```python
from build123d import *

# Parameters (mm, degrees)
ESQUISSE1_W                     = 250
ESQUISSE1_H                     = 400
BOSS_EXTRU_1_DEPTH              = 10
ESQUISSE2_R                     = 13.5
ENL_V_MAT_EXTRU_1_DEPTH         = 237.061432682
CHANFREIN1_SIZE                 = 3
TROU_TARAUD_M51_D               = 4.2
TROUS_DE_CENTRAGE_4_0MM2_D      = 4
TROUS_DE_CENTRAGE_6_0MM2_D      = 6
D_GAGEMENT_M41_D                = 4.5
R_P_TITION_LIN_AIRE1_COUNT      = 2
R_P_TITION_LIN_AIRE1_PITCH      = 120
R_P_TITION_LIN_AIRE1_COUNT_DIR2 = 2
R_P_TITION_LIN_AIRE1_PITCH_DIR2 = 340


with BuildPart() as part:
    # Esquisse1 → Boss.-Extru.1 (new body)
    with BuildSketch(Plane.XY):
        Rectangle(ESQUISSE1_W, ESQUISSE1_H)
    extrude(amount=BOSS_EXTRU_1_DEPTH)

    # Esquisse2 → Enlèv. mat.-Extru.1 (cut, through all)
    with BuildSketch(Plane(origin=(0, 0, 0), x_dir=(-1, 0, 0), z_dir=(0, 0, -1))):
        Circle(ESQUISSE2_R)
    extrude(amount=-ENL_V_MAT_EXTRU_1_DEPTH, mode=Mode.SUBTRACT)

    # Chanfrein1
    chanfrein1_edges = [part.edges().sort_by_distance(p)[0] for p in [
        (125, -200, 5),
        (-125, -200, 5),
        (-125, 200, 5),
        (125, 200, 5),
    ]]
    chamfer(chanfrein1_edges, length=CHANFREIN1_SIZE)

    # Trou taraudé M51 (through all)
    with Locations(Plane.XY.offset(10)):
        with Locations((-72.698486264, -161.07971462), (-72.698486264, -181.838730229), (-111.937151978, -181.838730229), (-111.937151978, -161.07971462)):
            Hole(TROU_TARAUD_M51_D / 2)

    # Trous de centrage Ø4.0mm2 (through all)
    with Locations(Plane.XY.offset(10)):
        with Locations((-93.86308218, -161.07971462), (-93.86308218, -181.838730229)):
            Hole(TROUS_DE_CENTRAGE_4_0MM2_D / 2)

    # Trous de centrage Ø6.0mm2 (through all)
    with Locations(Plane.XY.offset(10)):
        with Locations((16.357059687, 37.86831259), (37.86831259, -16.357059687), (-16.357059687, -37.86831259), (-37.86831259, 16.357059687)):
            Hole(TROUS_DE_CENTRAGE_6_0MM2_D / 2)

    # Dégagement M41 (through all)
    with Locations(Plane(origin=(0, 0, 0), x_dir=(-1, 0, 0), z_dir=(0, 0, -1))):
        with Locations((28, -187), (28, -157), (53, -157), (53, -187)):
            d_gagement_m41 = Hole(D_GAGEMENT_M41_D / 2)

    # Répétition linéaire1: D_gagement M41 2 × 2
    with Locations(*[(i * R_P_TITION_LIN_AIRE1_PITCH, j * R_P_TITION_LIN_AIRE1_PITCH_DIR2, 0) for i in range(R_P_TITION_LIN_AIRE1_COUNT) for j in range(R_P_TITION_LIN_AIRE1_COUNT_DIR2) if (i, j) != (0, 0)]):
        add(d_gagement_m41, mode=Mode.SUBTRACT)


solid = part.part
```
Here's how the part is built. I have some questions about the finished solid (model axes, mm). Round coordinates to 2 decimals unless told otherwise and drop trailing zeros. Answer as CSV lines item,"result". Start each with the question number.
1. I need wall thicknesses on probe 1 along Y at (x, z) = (-28, 4.5); probe 2 along X at (y, z) = (-157, 7.25); probe 3 along Y at (x, z) = (-112.5, 2.75). Which ranges of each line are inside material? Lowest first, please.
2. Thinking about a two-plate mould opening in Y: for faces 1 (the flat face through (-2, 200, 5)), 2 (the cylindrical face through (2.93, -13.18, 4.93)), 3 (the flat face through (-125, -3, 5)), which applies, released by +Y, released by -Y, zero draft, split by the parting line, or undercut?
3. I'm going to push flat-ended pins straight in: pin 1 Ø3.5 at (x, y) = (-53, 153) entering from -Z; pin 2 Ø6.5 at (x, y) = (-111.94, -161.08) entering from -Z. Where does each tip first touch, or does it pass through?
Check result:
1,probe 1,"y = -200 to -189.25, -184.75 to -159.25, -154.75 to 150.75, 155.25 to 180.75, 185.25 to 200"
1,probe 2,"x = -125 to -55.25, -50.75 to -30.25, -25.75 to 64.75, 69.25 to 89.75, 94.25 to 125"
1,probe 3,"y = -200 to -183.86, -179.82 to -163.1, -159.06 to 200"
2,face 1,"released by +Y"
2,face 2,"undercut"
2,face 3,"zero draft"
3,pin 1,"passes through"
3,pin 2,"stops at z = 0"
